Can you work these out from the model? Positions are in its coordinate system, mm. A direction names the side the tool comes from. Give positions to 0.01 mm unless a question says otherwise; leave off trailing zeros. Loops run counter-clockwise (first coordinate to the right, second up) from the corner with the lowest first, then second, coordinate; pieces in that order, holes last. Notation, with made-up numbers: (27.25, 28.5) - (86.25, 28.5) arc R23 ccw to (86.25, 59.5) - close; hole circle Ø3 at (-3.75, 1.5). An arc over 180 degrees is marked (long way). Answer as a JSON object with one key per item and string values.
Autodesk Inventor part; units mm, degrees
ref_plane "Work Plane2" through (30.0013, 0, 7.4992) normal (0, 0, -1) x (-1, 0, 0)
ref_plane "Work Plane3" through (-44.9987, 0, 7.4992) normal (0, 0, 1) x (1, 0, 0)
ref_plane "YZ Plane" through (0, 0, 0) normal (1, 0, 0) x (0, 1, 0)
sketch "Sketch1" plane through (0, 0, 0) normal (0, 1, 0) x (-1, 0, 0)
  line L0 (40, 90) -> (-40, 90)
  line L1 (-40, 90) -> (-40, -81.7795)
  line L2 (40, -41.5685) -> (40, 90)
  line L3 (40, 90) -> (-40, -90) construction
  line L4 (-40, 90) -> (40, -90) construction
  circle A0 centre (-0.0013, 54.9992) radius 5.1
  line L5 (23.4987, -16.5008) -> (-23.5013, -16.5008) construction
  line L6 (-23.5013, -16.5008) -> (-23.5013, -63.5008) construction
  line L7 (-23.5013, -63.5008) -> (23.4987, -63.5008) construction
  line L8 (23.4987, -63.5008) -> (23.4987, -16.5008) construction
  line L9 (23.4987, -16.5008) -> (-23.5013, -63.5008) construction
  line L10 (-23.5013, -16.5008) -> (23.4987, -63.5008) construction
  circle A1 centre (23.4987, -16.5008) radius 2.75
  circle A2 centre (23.4987, -63.5008) radius 2.75
  circle A3 centre (-23.5013, -16.5008) radius 2.75
  circle A4 centre (-23.5013, -63.5008) radius 2.75
  line L11 (-0.0013, -90.0008) -> (-0.0013, -80) construction
  line L12 (19.9987, -11.0008) -> (-20.0013, -11.0008) construction
  line L13 (-20.0013, -11.0008) -> (-20.0013, -69.0008) construction
  line L14 (-20.0013, -69.0008) -> (19.9987, -69.0008) construction
  line L15 (19.9987, -69.0008) -> (19.9987, -11.0008) construction
  line L16 (19.9987, -11.0008) -> (-20.0013, -69.0008) construction
  line L17 (-20.0013, -11.0008) -> (19.9987, -69.0008) construction
  line L18 (-29.0013, -60.0008) -> (28.9987, -60.0008) construction
  line L19 (28.9987, -60.0008) -> (28.9987, -20.0008) construction
  line L20 (28.9987, -20.0008) -> (-29.0013, -20.0008) construction
  line L21 (-29.0013, -20.0008) -> (-29.0013, -60.0008)
  line L22 (-29.0013, -60.0008) -> (28.9987, -20.0008) construction
  line L23 (28.9987, -60.0008) -> (-29.0013, -20.0008) construction
  line L24 (-0.0013, 54.9992) -> (102.5291, -47.5313) construction
  line L25 (-0.0013, 54.9992) -> (144.9987, 54.9992) construction
  line L26 (28.2843, 83.2843) -> (-28.2843, 26.7157) construction
  line L27 (-28.2843, 26.7157) -> (74.2462, -75.8148) construction
  line L28 (74.2462, -75.8148) -> (130.8148, -19.2462) construction
  line L29 (130.8148, -19.2462) -> (28.2843, 83.2843) construction
  line L30 (28.2843, 83.2843) -> (74.2462, -75.8148) construction
  line L31 (-28.2843, 26.7157) -> (130.8148, -19.2462) construction
  line L32 (74.2462, -75.8148) -> (14.1407, -135.9202)
  line L33 (14.1407, -135.9202) -> (-0.0014, -121.7781)
  line L34 (-0.0014, -121.7781) -> (-31.7795, -90)
  line L35 (74.2462, -75.8148) -> (40, -41.5685)
  line L36 (-31.7795, -90) -> (-40, -81.7795)
  line L37 (44.1935, -105.8675) -> (37.1224, -98.7964)
  line L38 (37.1224, -98.7964) -> (52.1488, -83.7701) construction
  line L39 (37.1224, -98.7964) -> (22.096, -113.8228) construction
  circle A5 centre (52.1488, -83.7701) radius 2.75
  circle A6 centre (22.096, -113.8228) radius 2.75
  line L40 (-0.0013, 54.9992) -> (-0.0013, -40.0008)
  circle A7 centre (-0.0013, -40.0008) radius 22.5
  point P0 (0, 0)
  point P1 (51.2639, 3.7339)
  dimension "d0" = 80
  dimension "d1" = 180
  dimension "d3" = 10.2
  dimension "d5" = 47
  dimension "d6" = 47
  dimension "d7" = 5.5
  dimension "d8" = 5.5
  dimension "d9" = 5.5
  dimension "d10" = 5.5
  dimension "d12" = 40
  dimension "d13" = 58
  dimension "d14" = 58
  dimension "d15" = 40
  dimension "d27" = 45
  dimension "d28" = 145
  dimension "d29" = 80
  dimension "d30" = 145
  dimension "d31" = 85.002
  dimension "d32" = 20
  dimension "d33" = 10
  dimension "d35" = 21.2505
  dimension "d36" = 21.2505
  dimension "d37" = 5.5
  dimension "d38" = 5.5
  dimension "d53" = 95
  dimension "d54" = 45
extrude "Plate3" add sketch "Sketch1" along normal blind 6
fillet "Fillet6" radius 5 4 edges at (-40, 3, -41.5685) (-74.2462, 3, -75.8148) (-14.1407, 3, -135.9202) (40, 3, -81.7795)
fillet "Fillet7" radius 40 2 edges at (40, 3, 90) (-40, 3, 90)
sketch "Sketch2" plane through (0, 0, 0) normal (0, -1, 0) x (1, 0, 0)
  circle A0 centre (0.0013, 54.9992) radius 5.1
  line L0 (0.0013, 54.9992) -> (0.0013, -40.0008) construction
  line L1 (0.0013, 7.4992) -> (55.0013, 7.4992) construction
  line L2 (0.0013, 7.4992) -> (-54.9987, 7.4992) construction
  line L3 (-29.9987, 7.4992) -> (30.0013, 7.4992) construction
  line L4 (-29.9987, 4.7492) -> (30.0013, 4.7492)
  line L5 (30.0013, 10.2492) -> (-29.9987, 10.2492)
  arc A1 (-29.9987, 10.2492) -> (-29.9987, 4.7492) centre (-29.9987, 7.4992) ccw
  arc A2 (30.0013, 4.7492) -> (30.0013, 10.2492) centre (30.0013, 7.4992) ccw
  point P0 (0, 0)
  dimension "d43" = 95
  dimension "d44" = 55
  dimension "d45" = 55
  dimension "d46" = 30
  dimension "d47" = 5.5
extrude "Extrusion1" cut sketch "Sketch2" against normal blind 10 contours A1 L5 A2 L4
ref_plane "Work Plane2" through (30.0013, 0, 7.4992) normal (0, 0, -1) x (-1, 0, 0)
sketch "Sketch3" plane through (0, 0, 0) normal (0, -1, 0) x (1, 0, 0)
  line L0 (-29.9987, 4.7492) -> (30.0013, 4.7492) construction
  line L1 (0.0013, 4.7492) -> (0.0013, 10.2492) construction
  line L2 (30.0013, 10.2492) -> (-29.9987, 10.2492) construction
  point P0 (0, 0)
sketch "Sketch4" plane through (0, 0, 0) normal (0, -1, 0) x (1, 0, 0)
  line L0 (-29.9987, 4.7492) -> (30.0013, 4.7492)
  line L1 (0.0013, 4.7492) -> (0.0013, 10.2492)
  line L2 (30.0013, 10.2492) -> (-29.9987, 10.2492)
  line L3 (-59.9987, 19.9992) -> (60.0013, 19.9992)
  line L4 (60.0013, 19.9992) -> (60.0013, -5.0008)
  line L5 (60.0013, -5.0008) -> (-59.9987, -5.0008)
  line L6 (-59.9987, -5.0008) -> (-59.9987, 19.9992)
  line L7 (-59.9987, 19.9992) -> (60.0013, -5.0008) construction
  line L8 (60.0013, 19.9992) -> (-59.9987, -5.0008) construction
  line L9 (-29.9987, 7.4992) -> (30.0013, 7.4992) construction
  line L10 (-29.9987, 4.7492) -> (30.0013, 4.7492)
  line L11 (30.0013, 10.2492) -> (-29.9987, 10.2492)
  arc A0 (-29.9987, 10.2492) -> (-29.9987, 4.7492) centre (-29.9987, 7.4992) ccw
  arc A1 (30.0013, 4.7492) -> (30.0013, 10.2492) centre (30.0013, 7.4992) ccw
  point P0 (0, 0)
  point P1 (0.0013, 7.4992)
  dimension "d56" = 120
  dimension "d57" = 25
sheet face with bend "Face4" sketch "Sketch4" thickness 6 toward (0, 1, 0) bend radius 6
bend "Bend1"
fillet "Fillet11" radius 9.75 4 edges at (60.0013, 3, -5.0008) (60.0013, 3, 19.9992) (-59.9987, 3, -5.0008) (-59.9987, 3, 19.9992)
sketch "Sketch5" plane through (0, 0, 0) normal (0, -1, 0) x (1, 0, 0)
  line L0 (-29.9987, 4.7492) -> (30.0013, 4.7492)
  line L1 (0.0013, 4.7492) -> (0.0013, 10.2492)
  line L2 (30.0013, 10.2492) -> (-29.9987, 10.2492)
  line L3 (-44.9987, 7.4992) -> (45.0013, 7.4992) construction
  line L4 (-44.9987, 4.7492) -> (45.0013, 4.7492)
  line L5 (45.0013, 10.2492) -> (-44.9987, 10.2492)
  arc A0 (-44.9987, 10.2492) -> (-44.9987, 4.7492) centre (-44.9987, 7.4992) ccw
  arc A1 (45.0013, 4.7492) -> (45.0013, 10.2492) centre (45.0013, 7.4992) ccw
  point P0 (0, 0)
  point P1 (0.0013, 7.4992)
  dimension "d64" = 45
  dimension "d65" = 5.5
extrude "Extrusion2" cut sketch "Sketch5" against normal blind 10
fillet "Fillet12" radius 9.75 4 edges at (40, 3, -5.0008) (-40, 3, -5.0008) (-40, 3, 19.9992) (40, 3, 19.9992)
sketch "Sketch6" plane through (0, 0, 0) normal (0, -1, 0) x (1, 0, 0)
  arc A0 (40, 29.7492) -> (49.75, 19.9992) centre (49.75, 29.7492) ccw
  arc A1 (-49.75, 19.9992) -> (-40, 29.7492) centre (-49.75, 29.7492) ccw
  line L0 (49.75, 19.9992) -> (-49.75, 19.9992)
  arc A2 (60.0013, 10.2492) -> (50.2513, 19.9992) centre (50.2513, 10.2492) ccw
  line L1 (50.2513, 19.9992) -> (-50.2487, 19.9992)
  line L2 (-50.2487, 19.9992) -> (-50.2487, 91.8023)
  line L3 (-50.2487, 91.8023) -> (50.2513, 91.8023)
  line L4 (50.2513, 91.8023) -> (50.2513, 19.9992)
  point P0 (0, 0)
extrude "Extrusion3" cut sketch "Sketch6" against normal through all
ref_plane "Work Plane3" through (-44.9987, 0, 7.4992) normal (0, 0, 1) x (1, 0, 0)
equation "\"d39\" = Thickness"
equation "\"BendRadius\" = Thickness"
equation "\"BendReliefWidth\" = Thickness"
equation "\"BendReliefDepth\" = 0.5 * Thickness"
equation "\"CornerReliefSize\" = 4 * Thickness"
equation "\"MinimumRemnant\" = 2 * Thickness"
equation "\"TransitionRadius\" = BendRadius"
equation "\"JacobiRadiusSize\" = BendRadius"
equation "\"GapSize\" = Thickness"
properties part number "NEMA23MountPlatev2" material "Aluminum 6061"
1) I need wall thicknesses on L1, parallel to Z at x = 5, y = 0.65; L2, parallel to Z at x = -43, y = 0.95; L3, parallel to Z at x = -23, y = 5.6. Which ranges of each line are inside material? Lowest first, please.
Check sheet entries:
{"L1": "-116.78 to -61.94, -18.06 to 4.75, 10.25 to 20", "L2": "-107.06 to -44.57, -7.72 to 4.75, 10.25 to 20", "L3": "-127.06 to -116.42, -111.23 to -66.21, -60.8 to -19.21, -13.8 to 4.75, 10.25 to 20"}
2) Imagine slicing it at B-B on x = 32. Write out the boundary of the cut face in (y, z).
Check sheet entries:
{"outline": "(0, -89.78) - (6, -89.78) - (6, 4.75) - (0, 4.75) - close; (0, 10.25) - (6, 10.25) - (6, 20) - (0, 20) - close"}
3) Imagine slicing it at D-D on x = 12. Write out the boundary of the cut face in (y, z), and give its area (3 significant figures).
Check sheet entries:
{"outline": "(0, -109.78) - (6, -109.78) - (6, -59.03) - (0, -59.03) - close; (0, -20.97) - (6, -20.97) - (6, 4.75) - (0, 4.75) - close; (0, 10.25) - (6, 10.25) - (6, 20) - (0, 20) - close", "area": "517 mm2"}
4) Imagine slicing it at A-A on z = -46.5. Write out the boundary of the cut face in (x, y), and give its area (3 significant figures).
Check sheet entries:
{"outline": "(-44.93, 0) - (-21.54, 0) - (-21.54, 6) - (-44.93, 6) - close; (21.54, 0) - (40, 0) - (40, 6) - (21.54, 6) - close", "area": "251 mm2"}
5) Imagine slicing it at C-C on y = 2. Give the number of separate pieces and of enclosed holes in the cut face, and give its area (3 significant figures).
Check sheet entries:
{"separate pieces": "1", "enclosed holes": "8", "area": "10,500 mm2"}
6) If we mould it in two halves opening along Z, with no side actions, what happens to faces 1 (the flat face through (1, 3, 10.249)), 2 (the cylindrical face through (-40.37, 3.04, -41.39)), 3 (the flat face through (-1, 3, 19.999)), 4 (the flat face through (40, 3, -47))? For each: released by +Z, released by -Z, zero draft, split by the parting line, or undercut.
Check sheet entries:
{"face 1": "undercut", "face 2": "undercut", "face 3": "released by +Z", "face 4": "zero draft"}
7) Which directions (+Z, -Z, +X, -X, +Y, -Y) give clear straight access to the entire face, cutting with the end or side of a thin tool? Please do faces 5 (the cylindrical face through (47.75, 2.96, 7.44)), 6 (the flat face through (-40, 3, -27)), 7 (the cylindrical face through (57.07, 3.04, 17.22)).
Check sheet entries:
{"face 5": "+Y, -Y", "face 6": "-X, +Y, -Y", "face 7": "+Z, +X, +Y, -Y"}
8) I'm going to push flat-ended pins straight in: P1, Ø3.5, axis at x = 23.5, z = -16.5, coming from the -Y side; P2, Ø6.5, axis at x = -22.1, z = -113.82, coming from the -Y side; P3, Ø1.8, axis at y = 4, z = -31, coming from the -X side; P4, Ø1.5, axis at y = 3, z = -97, coming from the -X side. Where does each tip first touch, or does it pass through?
Check sheet entries:
{"P1": "through", "P2": "y = 0", "P3": "x = -40", "P4": "x = -53.81"}
